from build123d import *

# Parameters (mm, degrees)
SKETCH_W        = 76
SKETCH_H        = 151
PAD_DEPTH       = 28
THICKNESS_T     = 1.3
SKETCH001_W     = 55
SKETCH001_H     = 13
POCKET_DEPTH    = 5
SKETCH002_W     = 21
SKETCH002_H     = 13
POCKET001_DEPTH = 5
SKETCH003_W     = 45
SKETCH003_H     = 15
POCKET002_DEPTH = 5


with BuildPart() as part:
    # Sketch → Pad (new body)
    with BuildSketch(Plane.XY):
        Rectangle(SKETCH_W, SKETCH_H)
    extrude(amount=PAD_DEPTH)

    # Thickness
    thickness_openings = [part.faces().sort_by_distance(p)[0] for p in [
        (0, 0, 28),
    ]]
    offset(amount=THICKNESS_T, openings=thickness_openings)

    # Sketch001 (on Face12 of Thickness) → Pocket (cut)
    with BuildSketch(Plane.XZ.offset(76.8)):
        with Locations((0, 10.5)):
            Rectangle(SKETCH001_W, SKETCH001_H)
    extrude(amount=-POCKET_DEPTH, mode=Mode.SUBTRACT)

    # Sketch002 (on Face11 of Pocket) → Pocket001 (cut)
    with BuildSketch(Plane(origin=(-39.3, 0, 0), x_dir=(0, -1, 0), z_dir=(-1, 0, 0))):
        with Locations((-49, 13.5)):
            Rectangle(SKETCH002_W, SKETCH002_H)
    extrude(amount=-POCKET001_DEPTH, mode=Mode.SUBTRACT)

    # Sketch003 (on Face11 of Pocket001) → Pocket002 (cut)
    with BuildSketch(Plane.YZ.offset(39.3)):
        with Locations((38, 13.5)):
            Rectangle(SKETCH003_W, SKETCH003_H)
    extrude(amount=-POCKET002_DEPTH, mode=Mode.SUBTRACT)


solid = part.part
Can you work these out from the model? Positions are in its coordinate system, mm. A direction names the side the tool comes from. Give positions to 0.01 mm unless a question says otherwise; leave off trailing zeros. Write each loop counter-clockwise with the first axis right and the second up, starting at its lowest first coordinate (ties: lowest second). Pieces come first, ordered by that corner, then holes. Notation, with made-up numbers: (-5.5, 85) -> (36.5, 85) arc R27 ccw to (36.5, 113) -> close; hole circle Ø9 at (-39.75, 63.5). An arc over 180 degrees is marked (long way). Answer as a JSON object with one key per item and string values. Group by question number.
Item 1: Suppose I cut it at C-C (z = 26). Please give me the cut outline in (x, y), plus the area to 3 significant figures.
Item 2: I'm going to push flat-ended pins straight in: P1, Ø0.6, axis at x = -39, z = 16.5, coming from the -Y side; P2, Ø3, axis at y = 38, z = 16.5, coming from the +X side; P3, Ø8, axis at x = -16, z = 12.5, coming from the -Y side. Where does each tip first touch, or does it pass through?
Item 3: Suppose I cut it at D-D (x = 34). Please give me the cut outline in (y, z), plus the area to 3 significant figures.
Item 4: Suppose I cut it at A-A (z = 9.25). Please give me the cut outline in (x, y).
Item 5: We'd pull the mould along Y, two halves only. Please class faces 1 (the face through (39.3, -1, 14)), 2 (the face through (-1, -75.5, 20)), 3 (the face through (-1, -76.8, 20)): +Y half, -Y half, draft (parallel to the pull), parting line (faces both ways), or undercut.
Item 6: For faces 4 (the face through (-1, 1, -1.3)), 5 (the face through (-1, 75.5, 14)), which set-ups out of +Z, -Z, +X, -X, +Y, -Y let a thin tool reach every point of the face, with its end or its side?
Item 7: Please list where these lines run through material, in increasing order: line 1 (Y direction, x = 2, z = 23.5); line 2 (X direction, y = 60, z = 25); line 3 (Z direction, x = 22.5, y = -47). Write a range as [from, to].
Item 8: Suppose I cut it at B-B (x = 11.5). Please give me the cut outline in (y, z), plus the area to 3 significant figures.
Findings:
{
 "1": {"outline": "(-39.3, -75.5) arc R1.3 ccw to (-38, -76.8) -> (38, -76.8) arc R1.3 ccw to (39.3, -75.5) -> (39.3, 75.5) arc R1.3 ccw to (38, 76.8) -> (-38, 76.8) arc R1.3 ccw to (-39.3, 75.5) -> close; hole (-38, -75.5) -> (38, -75.5) -> (38, 75.5) -> (-38, 75.5) -> close", "area": "596 mm²"},
 "2": {"P1": "stops at y = -76.6", "P2": "stops at x = -38", "P3": "stops at y = 75.5"},
 "3": {"outline": "(-76.8, 0) arc R1.3 ccw to (-75.5, -1.3) -> (75.5, -1.3) arc R1.3 ccw to (76.8, 0) -> (76.8, 28) -> (75.5, 28) -> (75.5, 0) -> (-75.5, 0) -> (-75.5, 28) -> (-76.8, 28) -> close", "area": "272 mm²"},
 "4": {"outline": "(-39.3, -75.5) arc R1.3 ccw to (-38, -76.8) -> (-27.5, -76.8) -> (-27.5, -75.5) -> (-38, -75.5) -> (-38, 38.5) -> (-39.3, 38.5) -> close; (-39.3, 59.5) -> (-38, 59.5) -> (-38, 75.5) -> (38, 75.5) -> (38, 60.5) -> (39.3, 60.5) -> (39.3, 75.5) arc R1.3 ccw to (38, 76.8) -> (-38, 76.8) arc R1.3 ccw to (-39.3, 75.5) -> close; (27.5, -76.8) -> (38, -76.8) arc R1.3 ccw to (39.3, -75.5) -> (39.3, 15.5) -> (38, 15.5) -> (38, -75.5) -> (27.5, -75.5) -> close"},
 "5": {"face 1": "draft", "face 2": "undercut", "face 3": "-Y half"},
 "6": {"face 4": "-Z, +X, -X, +Y, -Y", "face 5": "+Z"},
 "7": {"line 1": "y = [-76.8, -75.5], [75.5, 76.8]", "line 2": "x = [-39.3, -38], [38, 39.3]", "line 3": "z = [-1.3, 0]"},
 "8": {"outline": "(-76.8, 0) arc R1.3 ccw to (-75.5, -1.3) -> (75.5, -1.3) arc R1.3 ccw to (76.8, 0) -> (76.8, 28) -> (75.5, 28) -> (75.5, 0) -> (-75.5, 0) -> (-75.5, 4) -> (-76.8, 4) -> close; (-76.8, 17) -> (-75.5, 17) -> (-75.5, 28) -> (-76.8, 28) -> close", "area": "255 mm²"}
}
